Here's how the part is built. I have some questions about the finished solid (model axes, mm). Round coordinates to 2 decimals unless told otherwise and drop trailing zeros. Order: outer loops, then holes, each group sorted by start corner. A loop starts at its lowest first (then second) coordinate and runs counter-clockwise, first axis right, second up. Notation, with made-up numbers: (-18.5, 17) -> (33.5, 17) arc R16 ccw to (33.5, 38) -> close; hole circle Ø5 at (35, 84.5). An arc over 180 degrees is marked (long way). Use a Markdown table: item, result. Add a question column.
(1) I'm going to push flat-ended pins straight in: P1, Ø0.9, axis at x = 3.5, y = 20, coming from the +Z side; P2, Ø4.5, axis at y = 36, z = -4, coming from the +X side. Where does each tip first touch, or does it pass through?
(2) Thinking about a two-plate mould opening in X: for faces 1 (the face through (0, 20, -1)), 2 (the face through (2.11, 1.14, -4.89)), which applies, pulls with the +X half, pulls with the -X half, needs draft (parallel to the pull), parting line crosses it, or undercut?
(3) I want a section at A-A, the plane x = 3.75. Please give me the cut outline in (y, z), then the cut area to 3 significant figures.
(4) If I drill on probe 1 along Y at (x, z) = (1.6, -4); probe 2 along Z at (x, y) = (1.4, 4); probe 3 along Y at (x, z) = (0.5, -3.25), over which ranges is the centre line in solid material (lowest first)?
(5) I want a section at B-B, the plane y = 20. Give the number of separate pieces and of enclosed holes in the cut face, then the cut area to 3 significant figures.
from build123d import *

# Parameters (mm, degrees)
SKETCH1_W                  = 8
SKETCH1_H                  = 8
BOSS_EXTRUDE1_DEPTH        = 300
CUT_EXTRUDE1_DEPTH         = 301.213257535
SKETCH3_R                  = 2
CUT_EXTRUDE2_DEPTH         = 301.213257535
CHAMFER1_SIZE              = 0.3
CHAMFER2_SIZE              = 0.3
LPATTERN1_COUNT            = 19
LPATTERN1_PITCH            = 16
CHAMFER1_OF_LPATTERN1_SIZE = 0.3
SKETCH4_W                  = 8
SKETCH4_H                  = 260
CUT_EXTRUDE3_DEPTH         = 301.213257535


with BuildPart() as part:
    # Sketch1 → Boss-Extrude1 (new body)
    with BuildSketch(Plane(origin=(0, 0, 0), x_dir=(1, 0, 0), z_dir=(0, 1, 0))):
        with Locations((4, 4)):
            Rectangle(SKETCH1_W, SKETCH1_H)
    extrude(amount=BOSS_EXTRUDE1_DEPTH)

    # Sketch2 → Cut-Extrude1 (cut, through all)
    with BuildSketch(Plane.XZ):
        Polygon((5.652029979, 0), (2.008445554, 0), (2.008445554, -0.208206305), (2.54, -0.515099407), (1.673719601, -0.865099407), (2.54, -1.215099407), (1.673719601, -1.572712655), (2.54, -1.915099407), (1.673719601, -2.265099407), (2.54, -2.615099407), (1.673719601, -2.965099407), (2.54, -3.315099407), (1.673719601, -3.665099407), (2.54, -4.015099407), (1.673719601, -4.365099407), (2.54, -4.715099407), (1.673719601, -5.065099407), (2.54, -5.415099407), (1.673719601, -5.765099407), (2.54, -6.026380467), (2.54, -6.6), (5.46, -6.6), (5.46, -6.49878106), (6.106693316, -6.2375), (5.46, -5.8875), (6.106693316, -5.5375), (5.46, -5.1875), (6.106693316, -4.8375), (5.46, -4.4875), (6.106693316, -4.1375), (5.46, -3.7875), (6.106693316, -3.4375), (5.46, -3.0875), (6.106693316, -2.7375), (5.46, -2.3875), (6.106693316, -2.0375), (5.46, -1.6875), (6.106693316, -1.345113247), (5.46, -0.9875), (6.106693316, -0.6375), (5.652029979, -0.375), align=None)
    extrude(amount=-CUT_EXTRUDE1_DEPTH, mode=Mode.SUBTRACT)

    # Sketch3 → Cut-Extrude2 (cut, through all)
    with BuildSketch(Plane(origin=(8, 0, 0), x_dir=(0, 0, -1), z_dir=(1, 0, 0))):
        with Locations((4, 4)):
            Circle(SKETCH3_R)
    cut_extrude2 = extrude(amount=-CUT_EXTRUDE2_DEPTH, mode=Mode.SUBTRACT)

    # Chamfer1
    chamfer1_edges = [part.edges().sort_by_distance(p)[0] for p in [
        (0, 4, -2),
        (8, 4, -2),
    ]]
    chamfer(chamfer1_edges, length=CHAMFER1_SIZE)

    # Chamfer2
    chamfer2_edges = [part.edges().sort_by_distance(p)[0] for p in [
        (0, 150, -8),
        (8, 150, -8),
        (8, 150, 0),
        (0, 150, 0),
    ]]
    chamfer(chamfer2_edges, length=CHAMFER2_SIZE)

    # LPattern1: Cut-Extrude2 ×19
    with Locations(*[(0, i * LPATTERN1_PITCH, 0) for i in range(1, LPATTERN1_COUNT)]):
        add(cut_extrude2, mode=Mode.SUBTRACT)

    # Chamfer1 of LPattern1
    chamfer1_of_lpattern1_edges = [part.edges().sort_by_distance(p)[0] for p in [
        (0, 20, -2),
        (8, 20, -2),
        (0, 36, -2),
        (8, 36, -2),
        (0, 52, -2),
        (8, 52, -2),
        (0, 68, -2),
        (8, 68, -2),
        (0, 84, -2),
        (8, 84, -2),
        (0, 100, -2),
        (8, 100, -2),
        (0, 116, -2),
        (8, 116, -2),
        (0, 132, -2),
        (8, 132, -2),
        (0, 148, -2),
        (8, 148, -2),
        (0, 164, -2),
        (8, 164, -2),
        (0, 180, -2),
        (8, 180, -2),
        (0, 196, -2),
        (8, 196, -2),
        (0, 212, -2),
        (8, 212, -2),
        (0, 228, -2),
        (8, 228, -2),
        (0, 244, -2),
        (8, 244, -2),
        (0, 260, -2),
        (8, 260, -2),
        (0, 276, -2),
        (8, 276, -2),
        (0, 292, -2),
        (8, 292, -2),
    ]]
    chamfer(chamfer1_of_lpattern1_edges, length=CHAMFER1_OF_LPATTERN1_SIZE)

    # Sketch4 → Cut-Extrude3 (cut, through all)
    with BuildSketch(Plane(origin=(8, 0, 0), x_dir=(0, 0, -1), z_dir=(1, 0, 0))):
        with Locations((4, 170)):
            Rectangle(SKETCH4_W, SKETCH4_H)
    extrude(amount=-CUT_EXTRUDE3_DEPTH, mode=Mode.SUBTRACT)


solid = part.part
Taken from the geometry:
| question | item | result |
|---|---|---|
| 1 | P1 | stops at z = -6.6 |
| 1 | P2 | stops at x = 7.95 |
| 2 | face 1 | pulls with the -X half |
| 2 | face 2 | undercut |
| 3 | outline | (0, -8) -> (40, -8) -> (40, -6.6) -> (0, -6.6) -> close |
| 3 | area | 56.0 mm2 |
| 4 | probe 1 | y = 0 to 2, 6 to 18, 22 to 34, 38 to 40 |
| 4 | probe 2 | z = -8 to -6, -2 to 0 |
| 4 | probe 3 | y = 0 to 2.15, 5.85 to 18.15, 21.85 to 34.15, 37.85 to 40 |
| 5 | separate pieces | 3 |
| 5 | enclosed holes | 0 |
| 5 | area | 22.4 mm2 |
